Check sheet for the modelled part. Datum: model origin and axes. Units: mm. Give positions to 0.01 mm unless a question says otherwise; leave off trailing zeros. Order: outer loops, then holes, each group sorted by start corner. A loop starts at its lowest first (then second) coordinate and runs counter-clockwise, first axis right, second up.
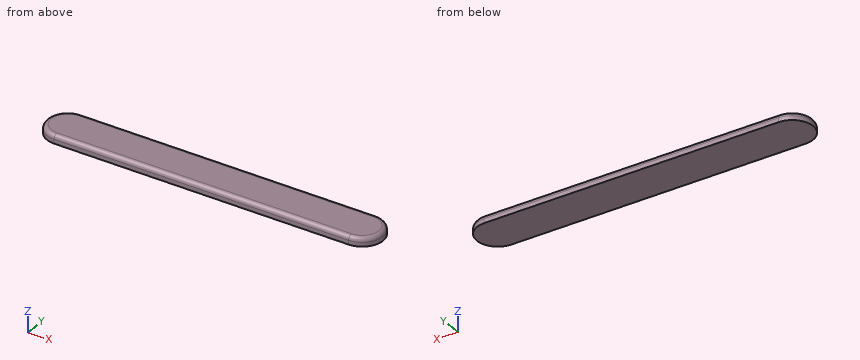
Autodesk Inventor part; units mm, degrees
ref_plane "YZ Plane" through (0, 0, 0) normal (1, 0, 0) x (0, 1, 0)
ref_plane "XZ Plane" through (0, 0, 0) normal (0, 1, 0) x (-1, 0, 0)
ref_plane "XY Plane" through (0, 0, 0) normal (0, 0, 1) x (1, 0, 0)
sketch "Sketch1" plane through (0, 0, 0) normal (0, 0, 1) x (1, 0, 0)
  line L0 (0, 0) -> (69.8, 0) construction
  line L1 (0, -4.9) -> (69.8, -4.9)
  line L2 (69.8, 4.9) -> (0, 4.9)
  arc A0 (0, 4.9) -> (0, -4.9) centre (0, 0) ccw
  arc A1 (69.8, -4.9) -> (69.8, 4.9) centre (69.8, 0) ccw
  point P0 (34.9, 0)
  dimension "d0" = 69.8
  dimension "d1" = 9.8
extrude "Extrusion1" add sketch "Sketch1" along normal blind 2
fillet "Fillet1" radius 1 4 edges at (-4.9, 0, 2) (34.9, -4.9, 2) (74.7, 0, 2) (34.9, 4.9, 2)
properties part number "foot"
(1) Thickness scan on L1, parallel to X at y = -0.25, z = 0.5; L2, parallel to Z at x = 32.5, y = 4; L3, parallel to X at y = -1, z = 0.3. Record the ranges inside material, lowest first.
(2) Sectioned sample at A-A (z = 0.7). Enter the section's corners in (x, y), plus the area to 3 significant figures.
(3) Sectioned sample at B-B (x = 59.5). Enter the section's corners in (y, z).
Values follow:
1. L1: x = -4.89 to 74.69
1. L2: z = 0 to 1.99
1. L3: x = -4.8 to 74.6
2. outline: (0, -4.9) - (69.8, -4.9) arc R4.9 ccw to (69.8, 4.9) - (0, 4.9) arc R4.9 ccw to start
2. area: 759 mm2
3. outline: (-4.9, 0) - (4.9, 0) - (4.9, 1) arc R1 ccw to (3.9, 2) - (-3.9, 2) arc R1 ccw to (-4.9, 1) - close
